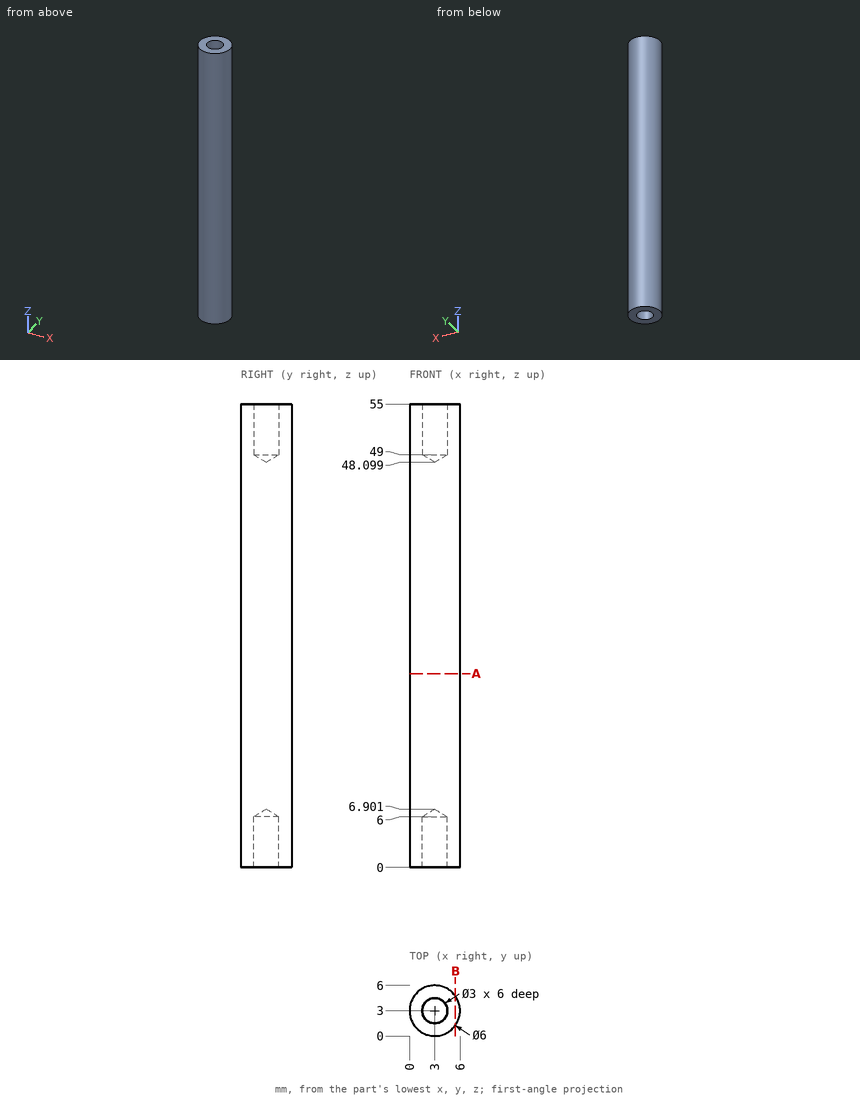
Print and shaded views of the part. All mm, measured from the part's lowest x, y and z. Give positions to 0.01 mm unless a question says otherwise; leave off trailing zeros. Loops run counter-clockwise (first coordinate to the right, second up) from the corner with the lowest first, then second, coordinate; pieces in that order, holes last. Notation, with made-up numbers: (7, -32) -> (22, -32) arc R25 cw to (22, -6) -> close; hole circle Ø6 at (43, 9). An arc over 180 degrees is marked (long way). Answer in a Markdown table with one row per item.
Item 1: Slice it at A-A on z = 23. Write the cut outline in (x, y).
Findings below:
| item | result |
|---|---|
| outline | circle Ø6 at (3, 3) |
Item 2: Probe line 1 along Y through (x, z) = (3, 50.5); line 2 along Y through (x, z) = (1.9, 4.5); line 3 along X through (y, z) = (2.85, 14). List the from-to ranges inside material, lowest first. Write a range as [from, to].
Findings below:
| item | result |
|---|---|
| line 1 | y = [0, 1.5], [4.5, 6] |
| line 2 | y = [0.21, 1.98], [4.02, 5.79] |
| line 3 | x = [0, 6] |
Item 3: Slice it at B-B on x = 5.45. Write the cut outline in (y, z).
Findings below:
| item | result |
|---|---|
| outline | (1.27, 0) -> (4.73, 0) -> (4.73, 55) -> (1.27, 55) -> close |
Item 4: Flat gauge pins, fed straight in: P1, Ø1.5, axis at y = 4.5, z = 8, coming from the +X side (1 decimal); P2, Ø2.5, axis at x = 3, y = 3, coming from the +Z side. Where does each tip first touch, or does it go through?
Findings below:
| item | result |
|---|---|
| P1 | stops at x = 5.9 |
| P2 | stops at z = 48.85 |
